from build123d import *

# Parameters (mm, degrees)
SKETCH1_W           = 190
SKETCH1_H           = 190
BOSS_EXTRUDE1_DEPTH = 10
CUT_EXTRUDE1_DEPTH  = 5
SKETCH3_W           = 61.021512422
SKETCH3_H           = 60
CUT_EXTRUDE2_DEPTH  = 139.021737418
SKETCH4_W           = 80
SKETCH4_H           = 80
CUT_EXTRUDE3_DEPTH  = 3
FILLET1_R           = 4
SHELL1_START        = -90
SHELL1_DEPTH        = 180
SHELL1_2_DEPTH      = 45
SHELL1_START_2      = 45
SHELL1_3_DEPTH      = 45


# Read off the part's stored shape, not the designer's step: Shell1
with BuildPart() as part:
    # Sketch1 → Boss-Extrude1 (new body)
    with BuildSketch(Plane(origin=(0, 0, 0), x_dir=(0, 0, -1), z_dir=(1, 0, 0))):
        with Locations((-5, 0)):
            Rectangle(SKETCH1_W, SKETCH1_H)
    extrude(amount=BOSS_EXTRUDE1_DEPTH)

    # Sketch2 → Cut-Extrude1 (cut)
    with BuildSketch(Plane.ZY):
        Polygon((36.5, -36.5), (36.5, 36.5), (25.709845909, 36.5), (5.209845909, 45.5), (-5.209845909, 45.5), (-25.709845909, 36.5), (-36.5, 36.5), (-36.5, -36.5), align=None)
    extrude(amount=-CUT_EXTRUDE1_DEPTH, mode=Mode.SUBTRACT)

    # Sketch3 → Cut-Extrude2 (cut, through all)
    with BuildSketch(Plane.ZY.offset(-5)):
        Rectangle(SKETCH3_W, SKETCH3_H)
    extrude(amount=-CUT_EXTRUDE2_DEPTH, mode=Mode.SUBTRACT)

    # Sketch4 → Cut-Extrude3 (cut)
    with BuildSketch(Plane(origin=(10, 0, 0), x_dir=(0, 0, -1), z_dir=(1, 0, 0))):
        Rectangle(SKETCH4_W, SKETCH4_H)
    extrude(amount=-CUT_EXTRUDE3_DEPTH, mode=Mode.SUBTRACT)

    # Fillet1
    fillet1_edges = [part.edges().sort_by_distance(p)[0] for p in [
        (10, 95, 5),
        (10, 0, 100),
        (5, 95, 100),
        (5, -95, 100),
    ]]
    fillet(fillet1_edges, radius=FILLET1_R)

    # Shell1 outline → Shell1 (cut)
    with BuildSketch(Plane(origin=(0, 0, 0), x_dir=(1, 0, 0), z_dir=(0, 1, 0)).offset(SHELL1_START)):
        Polygon((7, -45), (2, -45), (2, 45), (7, 45), (7, 85), (0, 85), (0, -95), (7, -95), align=None)
    extrude(amount=SHELL1_DEPTH, mode=Mode.SUBTRACT)

    # Shell1 2 outline → Shell1 2 (cut)
    with BuildSketch(Plane(origin=(0, 0, 0), x_dir=(1, 0, 0), z_dir=(0, 1, 0)).offset(SHELL1_START)):
        Polygon((2, -36.5), (2, -45), (7, -45), (7, 45), (2, 45), (2, 36.5), align=None)
    extrude(amount=SHELL1_2_DEPTH, mode=Mode.SUBTRACT)

    # Shell1 3 outline → Shell1 3 (cut)
    with BuildSketch(Plane(origin=(0, 0, 0), x_dir=(1, 0, 0), z_dir=(0, 1, 0)).offset(SHELL1_START_2)):
        Polygon((2, -36.5), (2, -45), (7, -45), (7, 45), (2, 45), (2, 36.5), align=None)
    extrude(amount=SHELL1_3_DEPTH, mode=Mode.SUBTRACT)


solid = part.part
Read the model definition and answer for the solid it produces. Units are mm, in the model's axes. A direction names the side the tool comes from. Coordinates: 2 decimals unless noted, no trailing zeros. Loops run counter-clockwise (first coordinate to the right, second up) from the corner with the lowest first, then second, coordinate; pieces in that order, holes last.
Q1. The part is cut by section A-A on y = 56.5. Write down the section's boundary in (x, z), and give its area (3 significant figures).
Q2. The part is cut by section C-C on x = 8.5. Write down the section's boundary in (y, z) (1 decimal).
Q3. The mould has two halves that part along Z. Classify faces 4 (the face through (3, -1, 95)), 5 (the face through (5, -95, 4)), 6 (the face through (3, -1, 100)), 7 (the face through (3.48, 40.81, -15.89)): +Z half, -Z half, draft (parallel to the pull), parting line (faces both ways), or undercut.
Q4. Which of the six approach directions +Z, -Z, +X, -X, +Y, -Y give full straight-line access (tool end or side, diameter ignored) to faces 1 (the face through (10, -1, 46)), 2 (the face through (4, -1, -45)), 3 (the face through (7, 1, 36))?
Q5. Consider probe 1 along Y at (x, z) = (4.5, 35); probe 2 along Y at (x, z) = (5.25, 31); probe 3 along Z at (x, y) = (1, 39). Determine where each line is inside the solid, lowest interval first.
Q6. The part is cut by section B-B on z = -60.5. Write down the section's boundary in (x, y).
Results below:
1. outline: (0, -90) - (10, -90) - (10, 96) arc R4 ccw to (6, 100) - (0, 100) - (0, 95) - (7, 95) - (7, -85) - (0, -85) - close
1. area: 637 mm2
2. outline: (-95, -90) - (94.1, -90) - (94.1, 96) arc R3.1 ccw to (91, 99.1) - (-93.5, 99.1) arc R4 ccw to (-95, 96) - close; hole (-40, -40) - (40, -40) - (40, 40) - (-40, 40) - close
3. face 4: undercut
3. face 5: draft
3. face 6: +Z half
3. face 7: undercut
4. face 1: +Z, -Z, +X, +Y, -Y
4. face 2: -X
4. face 3: +X
5. probe 1: y = -95 to -90, -45 to -36.5, 36.5 to 45, 90 to 95
5. probe 2: y = -95 to -90, -45 to 45, 90 to 95
5. probe 3: z = -90 to -85, 95 to 100
6. outline: (0, -95) - (10, -95) - (10, 91) arc R4 ccw to (6, 95) - (0, 95) - (0, 90) - (7, 90) - (7, -90) - (0, -90) - close
